For this review, take the finished solid that the model builds, in its own axes (mm). Face numbers are marked on the shaded views. A direction names the side the tool comes from. Coordinates: 2 decimals unless noted, no trailing zeros. Order: outer loops, then holes, each group sorted by start corner. A loop starts at its lowest first (then second) coordinate and runs counter-clockwise, first axis right, second up. Notation, with made-up numbers: (28.5, 15) - (33.5, 15) arc R28 ccw to (33.5, 49) - close; hole circle Ø1 at (-10, 73.25). An arc over 180 degrees is marked (long way). One line per item, written item: value. Start each with the question number.
(1) Clearance check with flat-ended pins moving along their axes: pin 1 (4 mm diameter, centred on y = 35.5, z = -13, fed in from +X); pin 2 (4 mm diameter, centred on x = -8, y = 20.5, fed in from -Z); pin 3 (4 mm diameter, centred on x = -8.5, z = -32, fed in from +Y). State where each tip first meets the part, or that it passes through.
(2) Consider section A-A on z = -51.5. Write out the cut boundary in (x, y), then the cut area to 3 significant figures.
(3) For the marked faces 1, 2 and 3, list the 3-axis set-ups (+Z, -Z, +X, -X, +Y, -Y) from which the entire face can be reached by the end or side of a thin tool; tool diameter is ignored.
(4) Consider section B-B on y = 21.5. Write out the cut boundary in (x, z).
(5) To check wall thickness, follow line 1 along X through (y, z) = (32.5, -9); line 2 along Z through (x, y) = (-6, 26); line 3 along Y through (x, z) = (-5.5, -6). State the ranges of each line that lie inside material, in increasing order.
Autodesk Inventor part; units mm, degrees
ref_plane "YZ Plane" through (0, 0, 0) normal (1, 0, 0) x (0, 1, 0)
ref_plane "XZ Plane" through (0, 0, 0) normal (0, 1, 0) x (-1, 0, 0)
ref_plane "XY Plane" through (0, 0, 0) normal (0, 0, 1) x (1, 0, 0)
sketch "Sketch1" plane through (0, 0, 0) normal (0, 1, 0) x (-1, 0, 0)
  line L0 (0, 0) -> (103.4, 0)
  line L1 (103.4, 0) -> (103.4, -62)
  line L2 (103.4, -62) -> (0, -62)
  line L3 (0, -62) -> (0, 0)
  dimension "d0" = 103.4
  dimension "d1" = 62
extrude "Extrusion1" add sketch "Sketch1" along normal blind 40
sketch "Sketch2" plane through (0, 0, -62) normal (0, 0, -1) x (-1, 0, 0)
  line L0 (103.4, 40) -> (0, 40)
  line L1 (51.7, 40) -> (90.7, 40)
  line L2 (103.4, 0) -> (103.4, 40)
  line L3 (90.7, 40) -> (103.4, 40)
  line L4 (103.4, 40) -> (103.4, 10.0001)
  line L5 (103.4, 10.0001) -> (90.7, 10.0001)
  line L6 (90.7, 10.0001) -> (90.7, 40)
  line L7 (51.7, 40) -> (51.7, 19.0962)
  line L8 (0, 10.0001) -> (12.7, 10.0001)
  line L9 (12.7, 10.0001) -> (12.7, 40)
  line L10 (0, 40) -> (103.4, 40)
  line L11 (0, 0) -> (0, 40)
  dimension "d4" = 39
extrude "Extrusion2" cut sketch "Sketch2" against normal blind 60
properties part number "RPS-120-12 power supply"
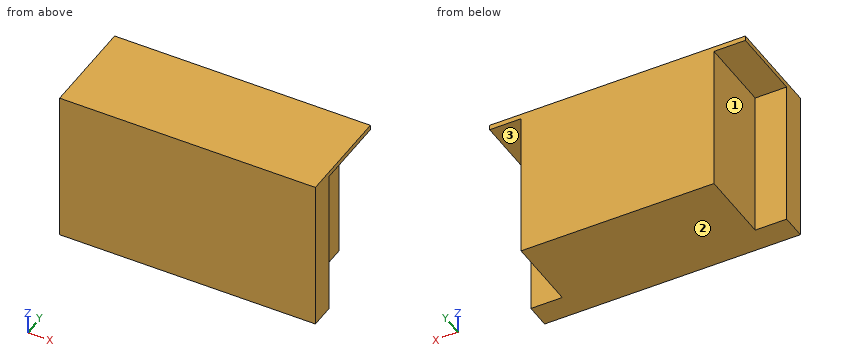
Geometry check:
1. pin 1: stops at x = -12.7
1. pin 2: stops at z = -2
1. pin 3: stops at y = 10
2. outline: (-103.4, 0) - (0, 0) - (0, 10) - (-12.7, 10) - (-12.7, 40) - (-90.7, 40) - (-90.7, 10) - (-103.4, 10) - close
2. area: 3,370 mm^2
3. face 1: -Z, -X, +Y
3. face 2: -Z, +X, -X, +Y, -Y
3. face 3: -Z, +X, +Y
4. outline: (-103.4, -2) - (-90.7, -2) - (-90.7, -62) - (-12.7, -62) - (-12.7, -2) - (0, -2) - (0, 0) - (-103.4, 0) - close
5. line 1: x = -90.7 to -12.7
5. line 2: z = -2 to 0
5. line 3: y = 0 to 10
